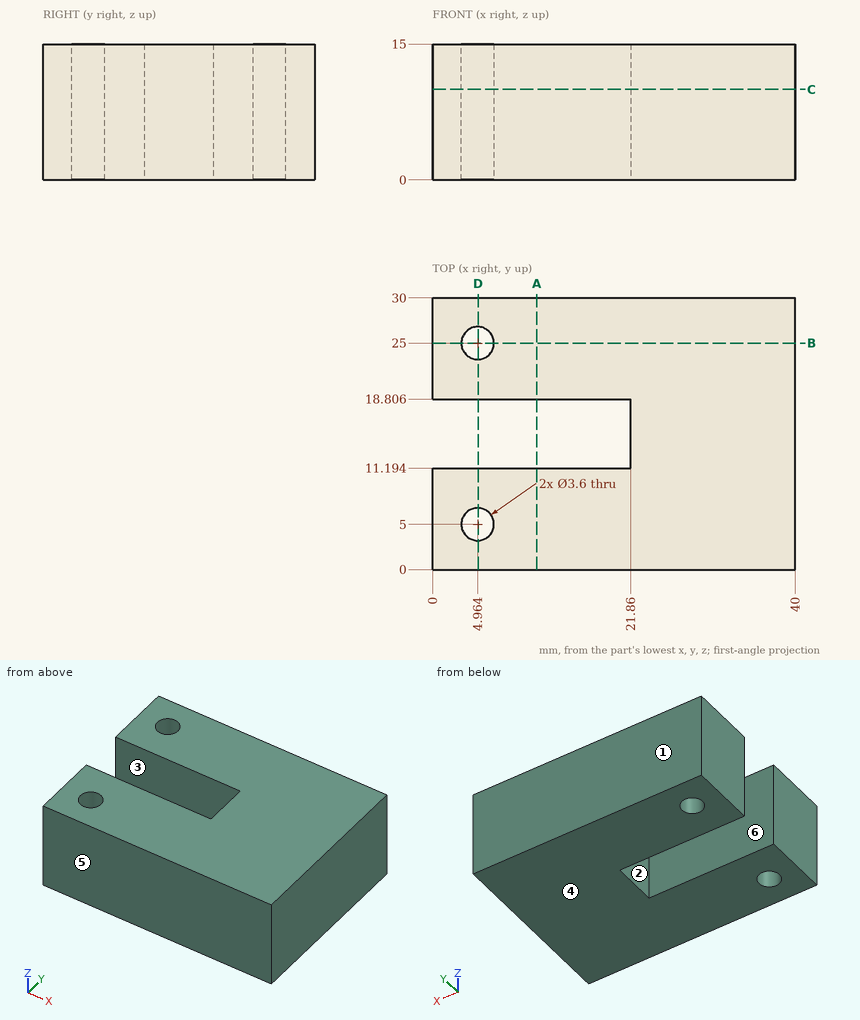
The drawing under review shows one solid part. Ordinate dimensions are in mm from its lowest x, y, z. A direction names the side the tool comes from. Round coordinates to 2 decimals unless told otherwise and drop trailing zeros. Write each loop counter-clockwise with the first axis right and the second up, starting at its lowest first coordinate (ties: lowest second). Pieces come first, ordered by that corner, then holes. Notation, with made-up numbers: (43, 1.5) -> (93, 1.5) arc R15 cw to (93, 20.5) -> close; hole circle Ø2 at (14, 81.25). An arc over 180 degrees is marked (long way). Put each result on its own line as item: value.
Q1. To check wall thickness, follow L1, parallel to Y at x = 2, z = 1.25; L2, parallel to X at y = 5.5, z = 2.5 (1 decimal); L3, parallel to Y at x = 5.5, z = 8. State the ranges of each line that lie inside material, in increasing order. Write a range as [from, to].
Determined:
L1: y = [0, 11.19], [18.81, 30]
L2: x = [0, 3.2], [6.7, 40]
L3: y = [0, 3.28], [6.72, 11.19], [18.81, 23.28], [26.72, 30]
Q2. The part is to be moulded in two halves that separate along Y. For the marked faces 1, 2, 3 and 4, say which applies: released by +Y, released by -Y, zero draft, split by the parting line, or undercut.
Determined:
face 1: released by +Y
face 2: undercut
face 3: undercut
face 4: zero draft
Q3. Consider section B-B on y = 25. State the section outline as (x, z) points, and give its area (3 significant figures).
Determined:
outline: (0, 0) -> (3.16, 0) -> (3.16, 15) -> (0, 15) -> close; (6.76, 0) -> (40, 0) -> (40, 15) -> (6.76, 15) -> close
area: 546 mm^2
Q4. Consider section A-A on x = 11.5. State the section outline as (y, z) points.
Determined:
outline: (0, 0) -> (11.19, 0) -> (11.19, 15) -> (0, 15) -> close; (18.81, 0) -> (30, 0) -> (30, 15) -> (18.81, 15) -> close
Q5. Consider section D-D on x = 5. State the section outline as (y, z) points, and give its area (3 significant figures).
Determined:
outline: (0, 0) -> (3.2, 0) -> (3.2, 15) -> (0, 15) -> close; (6.8, 0) -> (11.19, 0) -> (11.19, 15) -> (6.8, 15) -> close; (18.81, 0) -> (23.2, 0) -> (23.2, 15) -> (18.81, 15) -> close; (26.8, 0) -> (30, 0) -> (30, 15) -> (26.8, 15) -> close
area: 228 mm^2
Q6. Machinability: for the marked faces 5 and 6, which of the approach directions +Z, -Z, +X, -X, +Y, -Y give a long, thin tool a straight path to every point of the face, cutting with its end or side? Answer none if there is none.
Determined:
face 5: +Z, -Z, +X, -X, -Y
face 6: +Z, -Z, -X
Q7. Consider section C-C on z = 10. State the section outline as (x, y) points.
Determined:
outline: (0, 0) -> (40, 0) -> (40, 30) -> (0, 30) -> (0, 18.81) -> (21.86, 18.81) -> (21.86, 11.19) -> (0, 11.19) -> close; hole circle Ø3.6 at (4.96, 5); hole circle Ø3.6 at (4.96, 25)
